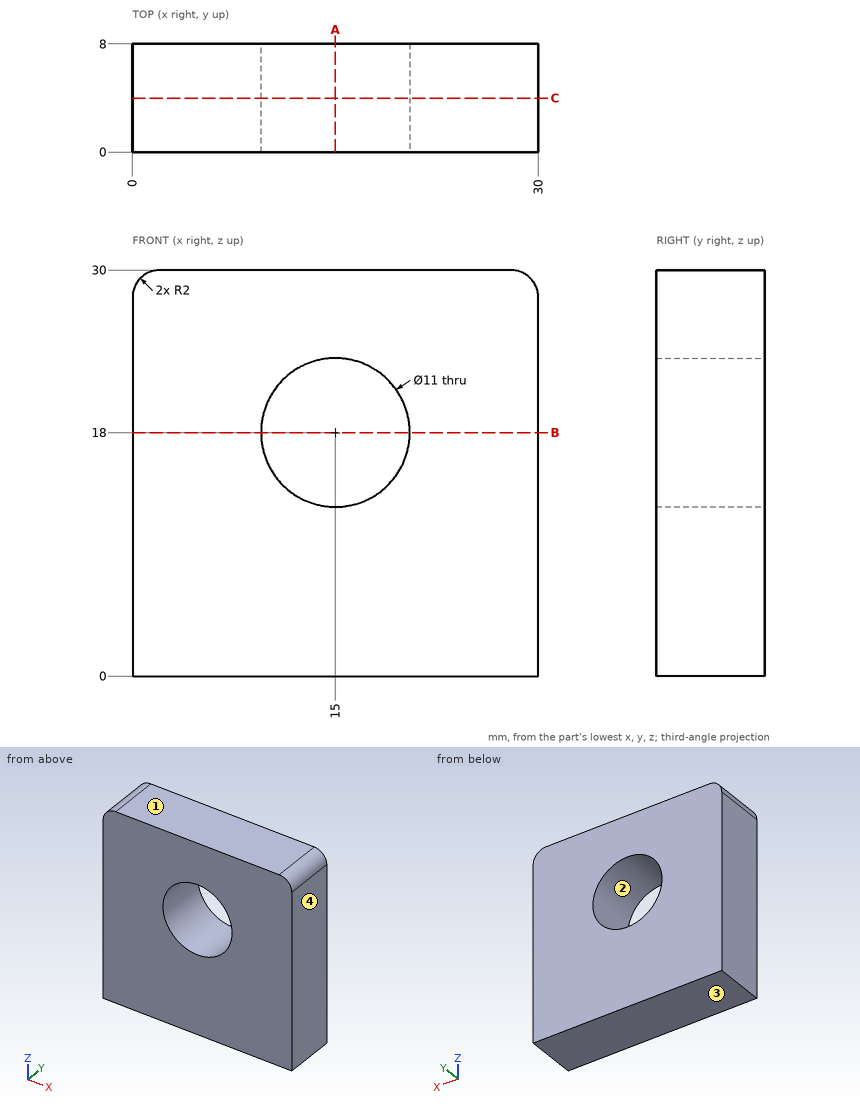
Answer from the drawing. Dimensions are ordinates in mm from the lowest x, y and z of the part. Coordinates: 2 decimals unless noted, no trailing zeros. Order: outer loops, then holes, each group sorted by start corner. A loop starts at its lowest first (then second) coordinate and runs counter-clockwise, first axis right, second up. Notation, with made-up numbers: M -37.75,42.25 L 12.25,42.25 A23 cw 12.25,66.25 Z; hole C 22.25,26.5 d2. An arc over 180 degrees is marked long. Put each result on its own line as item: value. Start each with the question number.
Item 1: Section C-C, the plane y = 4 is taken. Determine the outline of the cut face in (x, z).
Item 2: Consider probe 1 along Z at (x, y) = (15, 2.5); probe 2 along X at (y, z) = (7.75, 14.5); probe 3 along Z at (x, y) = (13, 0.75). Determine where each line is inside the solid, lowest interval first. Write a range as [from, to].
Item 3: Section B-B, the plane z = 18 is taken. Determine the outline of the cut face in (x, y).
Item 4: Section A-A, the plane x = 15 is taken. Determine the outline of the cut face in (y, z).
Item 5: The mould has two halves that part along Z. Classify the marked faces 1, 2, 3 and 4: +Z half, -Z half, draft (parallel to the pull), parting line (faces both ways), or undercut.
Computed:
1. outline: M 0,0 L 30,0 L 30,28 A2 ccw 28,30 L 2,30 A2 ccw 0,28 Z; hole C 15,18 d11
2. probe 1: z = [0, 12.5], [23.5, 30]
2. probe 2: x = [0, 10.76], [19.24, 30]
2. probe 3: z = [0, 12.88], [23.12, 30]
3. outline: M 0,0 L 9.5,0 L 9.5,8 L 0,8 Z; M 20.5,0 L 30,0 L 30,8 L 20.5,8 Z
4. outline: M 0,0 L 8,0 L 8,12.5 L 0,12.5 Z; M 0,23.5 L 8,23.5 L 8,30 L 0,30 Z
5. face 1: +Z half
5. face 2: undercut
5. face 3: -Z half
5. face 4: draft
